```python
from build123d import *

# Parameters (mm, degrees)
SKETCH1_W               = 44
SKETCH1_H               = 32
BOSS_EXTRUDE1_DEPTH     = 12
SKETCH2_W               = 24.5
SKETCH2_H               = 15.5
CUT_EXTRUDE1_DEPTH      = 7.75
FILLET1_R               = 7.75
CUT_EXTRUDE2_DEPTH      = 40.661851949
CUT_EXTRUDE2_DEPTH_BACK = 40.661851949
SKETCH4_R               = 2.75
SKETCH4_W               = 20
SKETCH4_H               = 10.5
CUT_EXTRUDE3_DEPTH      = 30.732137495
SKETCH5_W               = 5.5
SKETCH5_H               = 3
BOSS_EXTRUDE4_DEPTH     = 7
CHAMFER1_SIZE           = 7
SKETCH6_W               = 11.5
SKETCH6_H               = 7
CUT_EXTRUDE5_DEPTH      = 30.732137495
FILLET4_R               = 5.5
SKETCH7_W               = 10
SKETCH7_H               = 10
SKETCH7_R               = 2
BOSS_EXTRUDE5_DEPTH     = 5
CUT_EXTRUDE6_START      = -2
SKETCH8_R               = 2
CUT_EXTRUDE6_DEPTH      = 2
FILLET5_R               = 5
CUT_EXTRUDE7_START      = -4
SKETCH9_R               = 2.75
CUT_EXTRUDE7_DEPTH      = 4


with BuildPart() as part:
    # Sketch1 → Boss-Extrude1 (new body)
    with BuildSketch(Plane(origin=(0, 0, 0), x_dir=(0, 0, -1), z_dir=(1, 0, 0))):
        Rectangle(SKETCH1_W, SKETCH1_H)
    extrude(amount=BOSS_EXTRUDE1_DEPTH)

    # Sketch2 → Cut-Extrude1 (cut)
    with BuildSketch(Plane(origin=(0, 0, 0), x_dir=(0, 0, -1), z_dir=(1, 0, 0))):
        with Locations((0, -5.25)):
            Rectangle(SKETCH2_W, SKETCH2_H)
    extrude(amount=CUT_EXTRUDE1_DEPTH, mode=Mode.SUBTRACT)

    # Fillet1
    fillet1_edges = [part.edges().sort_by_distance(p)[0] for p in [
        (7.75, 2.5, 0),
        (7.75, -13, 0),
    ]]
    fillet(fillet1_edges, radius=FILLET1_R - 0.0001)  # a hair under: the kernel refuses the full size

    # Sketch3 → Cut-Extrude2 (cut, two sides: drawn at the far end of the back side and taken through both)
    with BuildSketch(Plane.XY.offset(-12.25).offset(-CUT_EXTRUDE2_DEPTH_BACK)):
        with BuildLine():
            ThreePointArc((0, -10.25), (3.535533906, -8.785533906), (5, -5.25))
            ThreePointArc((5, -5.25), (3.535533906, -1.714466094), (0, -0.25))
            Line((0, -0.25), (0, -10.25))
        make_face()
        with BuildLine():
            Line((0, -10.25), (0, -0.25))
            ThreePointArc((0, -0.25), (-5, -5.25), (0, -10.25))
        make_face()
    extrude(amount=CUT_EXTRUDE2_DEPTH + CUT_EXTRUDE2_DEPTH_BACK, mode=Mode.SUBTRACT)

    # Sketch4 → Cut-Extrude3 (cut, through all)
    with BuildSketch(Plane(origin=(12, 0, 0), x_dir=(0, 0, -1), z_dir=(1, 0, 0))):
        with Locations((-16, 10)):
            Circle(SKETCH4_R)
        with Locations((16, 10)):
            Circle(SKETCH4_R)
        with Locations((0, 10.75)):
            Rectangle(SKETCH4_W, SKETCH4_H)
    extrude(amount=-CUT_EXTRUDE3_DEPTH, mode=Mode.SUBTRACT)

    # Sketch5 → Boss-Extrude4 (add)
    with BuildSketch(Plane(origin=(12, 0, 0), x_dir=(0, 0, -1), z_dir=(1, 0, 0))):
        Polygon((-16, -3), (-16, 4.5), (-2.75, -3), align=None)
        Polygon((-2.75, -3), (-16, 4.5), (-2.75, 0), align=None)
        with Locations((0, -1.5)):
            Rectangle(SKETCH5_W, SKETCH5_H)
        Polygon((2.75, -3), (2.75, 0), (16, 4.5), align=None)
        Polygon((16, -3), (2.75, -3), (16, 4.5), align=None)
    extrude(amount=BOSS_EXTRUDE4_DEPTH)

    # Chamfer1
    chamfer1_edges = [part.edges().sort_by_distance(p)[0] for p in [
        (12, -3, 0),
    ]]
    chamfer(chamfer1_edges, length=CHAMFER1_SIZE - 0.0001)  # a hair under: the kernel refuses the full size

    # Sketch6 → Cut-Extrude5 (cut, through all)
    with BuildSketch(Plane(origin=(12, 0, 0), x_dir=(0, 0, -1), z_dir=(1, 0, 0))):
        with Locations((-7.25, -6.5)):
            Rectangle(SKETCH6_W, SKETCH6_H)
        with Locations((7.25, -6.5)):
            Rectangle(SKETCH6_W, SKETCH6_H)
    extrude(amount=CUT_EXTRUDE5_DEPTH, mode=Mode.SUBTRACT)

    # Fillet4
    fillet4_edges = [part.edges().sort_by_distance(p)[0] for p in [
        (6, 16, 22),
        (6, 16, -22),
    ]]
    fillet(fillet4_edges, radius=FILLET4_R)

    # Sketch7 → Boss-Extrude5 (add)
    with BuildSketch(Plane(origin=(0, 0, 0), x_dir=(0, 0, -1), z_dir=(1, 0, 0))):
        with Locations((0, -21)):
            Rectangle(SKETCH7_W, SKETCH7_H)
        with Locations((0, -21)):
            Circle(SKETCH7_R, mode=Mode.SUBTRACT)
    extrude(amount=BOSS_EXTRUDE5_DEPTH)

    # Sketch8 → Cut-Extrude6 (cut)
    with BuildSketch(Plane(origin=(5, 0, 0), x_dir=(0, 0, -1), z_dir=(1, 0, 0)).offset(CUT_EXTRUDE6_START)):
        Polygon((0, -24.175426481), (2.75, -22.58771324), (2.75, -19.41228676), (0, -17.824573519), (-2.75, -19.41228676), (-2.75, -22.58771324), align=None)
        with Locations((0, -21)):
            Circle(SKETCH8_R, mode=Mode.SUBTRACT)
    extrude(amount=CUT_EXTRUDE6_DEPTH, mode=Mode.SUBTRACT)

    # Fillet5
    fillet5_edges = [part.edges().sort_by_distance(p)[0] for p in [
        (2.5, -26, -5),
        (2.5, -26, 5),
    ]]
    fillet(fillet5_edges, radius=FILLET5_R - 0.0001)  # a hair under: the kernel refuses the full size

    # Sketch9 → Cut-Extrude7 (cut)
    # profile 1 of 2: a face of its own
    with BuildSketch(Plane.ZY.offset(CUT_EXTRUDE7_START)):
        Polygon((-16, 5.381197846), (-12, 7.690598923), (-12, 12.309401077), (-16, 14.618802154), (-20, 12.309401077), (-20, 7.690598923), align=None)
        with Locations(Location((-16, 10, 0), (0, 0, 180))):
            Circle(SKETCH9_R, mode=Mode.SUBTRACT)
    # profile 2 of 2: a face of its own
    with BuildSketch(Plane.ZY.offset(CUT_EXTRUDE7_START)):
        Polygon((16, 5.381197846), (20, 7.690598923), (20, 12.309401077), (16, 14.618802154), (12, 12.309401077), (12, 7.690598923), align=None)
        with Locations(Location((16, 10, 0), (0, 0, 180))):
            Circle(SKETCH9_R, mode=Mode.SUBTRACT)
    extrude(amount=CUT_EXTRUDE7_DEPTH, mode=Mode.SUBTRACT)


solid = part.part
```
The listing builds one solid part. Answer for the finished solid, in the listing's coordinates (mm). A direction names the side the tool comes from. Coordinates: 2 decimals unless noted, no trailing zeros. Loops run counter-clockwise (first coordinate to the right, second up) from the corner with the lowest first, then second, coordinate; pieces in that order, holes last. Notation, with made-up numbers: M 61.5,38.5 L 67.5,38.5 A17 ccw 67.5,64.5 Z; hole C -0.75,81 d5. An arc over 180 degrees is marked long. Answer as CSV lines item,"result". Start each with the question number.
(1) For faces 5 (the flat face through (3, -23, 1)), 6 (the flat face through (6, 11, 10)), 7 (the flat face through (15, -1, -16)), 8 (the flat face through (2.028, 6.552, 13.972)), determine the directions among +Z, -Z, +X, -X, +Y, -Y from which every point of the face is accessible in a straight line to the end or side of a thin tool.
(2) Given pin 1 (5 mm diameter, centred on y = -22, z = 2.5, fed in from +X); pin 2 (7.5 mm diameter, centred on x = 14, y = -6, fed in from -Z); pin 3 (5 mm diameter, centred on y = -21, z = 0, fed in from +X); pin 4 (7.5 mm diameter, centred on x = 16.5, y = -5, fed in from +Z), each flat-ended and moving along its own axis, determine where each tip first touches the part or whether it passes through.
(3) Find the intervals of material crossed by L1, parallel to Z at x = 10, y = 10; L2, parallel to Z at x = 4, y = -20; L3, parallel to Z at x = 10.5, y = 9, in increasing order. Write a range as [from, to].
(4) The mould has two halves that part along Z. Classify faces 1 (the flat face through (4, -21, -2.75)), 2 (the flat face through (5, -18.7, -2.2)), 3 (the flat face through (2.028, 6.552, -18.028)), 4 (the cylindrical face through (3, -24, 4)): pulls with the +Z half, pulls with the -Z half, needs draft (parallel to the pull), parting line crosses it, or undercut.
(5) The part is cut by section C-C (y = -9). Give the vertices of the cut face in (x, z).
(6) The part is cut by section A-A (x = 11.25). Give the vertices of the cut face in (y, z).
(7) The part is cut by section D-D (x = 15.75). Give the vertices of the cut face in (y, z).
Determined:
1,face 5,"+X"
1,face 6,"+X, -X, +Y"
1,face 7,"-Z, +X, +Y, -Y"
1,face 8,"-X"
2,pin 1,"x = 5"
2,pin 2,"z = -22"
2,pin 3,"x = 3"
2,pin 4,"z = 16"
3,L1,"[-22, -18.75], [-13.25, -10], [10, 13.25], [18.75, 22]"
3,L2,"[-5, -2.75], [2.75, 5]"
3,L3,"[-22, -18.56], [-13.44, -10], [10, 13.44], [18.56, 22]"
4,face 1,"undercut"
4,face 2,"needs draft"
4,face 3,"undercut"
4,face 4,"pulls with the +Z half"
5,outline,"M 3.31,-22 L 12,-22 L 12,-16 L 13,-16 L 13,-13 L 12,-13 L 12,-1.5 L 13,-1.5 L 13,1.5 L 12,1.5 L 12,13 L 13,13 L 13,16 L 12,16 L 12,22 L 3.31,22 L 3.31,12.25 L 6.78,12.25 L 6.78,-12.25 L 3.31,-12.25 Z"
6,outline,"M -16,-22 L 10.5,-22 A5.5 ccw 16,-16.5 L 16,-10 L 5.5,-10 L 5.5,10 L 16,10 L 16,16.5 A5.5 ccw 10.5,22 L -16,22 Z; hole C 10,-16 d5.5; hole C 10,16 d5.5"
7,outline,"M -6.25,-16 L 4.5,-16 L 0,-2.75 L 0,2.75 L 4.5,16 L -6.25,16 L -6.25,13 L -3,13 L -3,1.5 L -6.25,1.5 L -6.25,-1.5 L -3,-1.5 L -3,-13 L -6.25,-13 Z"
